Source: CAD feature listing. Evaluate the final solid. Frame: model axes, mm. Coordinates: 2 decimals unless noted, no trailing zeros. Loops run counter-clockwise (first coordinate to the right, second up) from the corner with the lowest first, then second, coordinate; pieces in that order, holes last. Notation, with made-up numbers: M 24,26 L 59,26 A19 cw 59,39 Z; hole C 14.25,-6.75 d5. An arc over 180 degrees is marked long. One line per question, with ' | ' between items. Start each with the question number.
1. Section query A-A, the plane x = 31.75. Output: boundary loops of the cut face in (y, z) (3 decimals).
2. Ray query, probe 1 along X at (y, z) = (5.5, -19.05) (3 decimals); probe 2 along X at (y, z) = (5, 19); probe 3 along Z at (x, y) = (-31, 10). Return the intervals inside material, ascending.
3. Mould query, pull axis Z, two halves, no side actions, for faces 1 (the flat face through (0, 50.8, 0)), 2 (the flat face through (-1, 6, 31.75)), 3 (the cylindrical face through (-34.85, 6.39, -19.74)). Classes: pulls with the +Z half, pulls with the -Z half, needs draft (parallel to the pull), parting line crosses it, or undercut.
4. Pin query (flat end, axial travel): P1, Ø10.5, axis at x = 31.75, z = -19.05, coming from the -Y side; P2, Ø12, axis at y = 28.5, z = 3, coming from the -X side; P3, Ø1, axis at x = 8.5, y = 19.5, coming from the +Z side; P4, Ø7.5, axis at x = -31.75, z = 19.05, coming from the +Y side. Return the tip coordinate at first contact, or that it passes through.
5. Section query D-D, the plane z = 0. Output: boundary loops of the cut face in (x, y).
6. Section query C-C, the plane y = 7. Output: boundary loops of the cut face in (x, z) (3 decimals), and give its area (3 significant figures).
7. Section query B-B, the plane z = 19.05. Output: boundary loops of the cut face in (x, y) (3 decimals).
```python
from build123d import *

# Parameters (mm, degrees)
SKETCH1_W           = 101.6
SKETCH1_H           = 63.5
SKETCH1_R           = 3.175
SKETCH1_R_2         = 3.349234597
BOSS_EXTRUDE1_DEPTH = 12.7
SKETCH2_R           = 12.7
BOSS_EXTRUDE2_DEPTH = 38.1
CHAMFER1_SIZE       = 3.81
FILLET1_R           = 5.08
CHAMFER2_SIZE       = 0.254


with BuildPart() as part:
    # Sketch1 → Boss-Extrude1 (new body)
    with BuildSketch(Plane(origin=(0, 0, 0), x_dir=(1, 0, 0), z_dir=(0, 1, 0))):
        Rectangle(SKETCH1_W, SKETCH1_H)
        with Locations(Location((-31.75, 19.05, 0), (0, 0, 270))):
            Circle(SKETCH1_R, mode=Mode.SUBTRACT)
        with Locations(Location((-31.75, -19.05, 0), (0, 0, 270))):
            Circle(SKETCH1_R, mode=Mode.SUBTRACT)
        with Locations(Location((31.75, -19.05, 0), (0, 0, 270))):
            Circle(SKETCH1_R, mode=Mode.SUBTRACT)
        with Locations(Location((31.75, 19.05, 0), (0, 0, 270))):
            Circle(SKETCH1_R_2, mode=Mode.SUBTRACT)
    extrude(amount=BOSS_EXTRUDE1_DEPTH)

    # Sketch2 → Boss-Extrude2 (add)
    with BuildSketch(Plane(origin=(0, 12.7, 0), x_dir=(1, 0, 0), z_dir=(0, 1, 0))):
        with Locations(Location((0, 0, 0), (0, 0, 90))):
            Circle(SKETCH2_R)
    extrude(amount=BOSS_EXTRUDE2_DEPTH)

    # Chamfer1
    chamfer1_edges = [part.edges().sort_by_distance(p)[0] for p in [
        (0, 12.7, 12.7),
    ]]
    chamfer(chamfer1_edges, length=CHAMFER1_SIZE)

    # Fillet1
    fillet1_edges = [part.edges().sort_by_distance(p)[0] for p in [
        (50.8, 6.35, 31.75),
        (-50.8, 6.35, 31.75),
        (-50.8, 6.35, -31.75),
        (50.8, 6.35, -31.75),
    ]]
    fillet(fillet1_edges, radius=FILLET1_R)

    # Chamfer2
    chamfer2_edges = [part.edges().sort_by_distance(p)[0] for p in [
        (-31.75, 0, 15.875),
        (-31.75, 0, -22.225),
        (31.75, 0, 15.875),
        (31.75, 0, -22.399234597),
        (0, 0, 31.75),
        (50.8, 0, 0),
        (-50.8, 0, 0),
        (0, 0, -31.75),
        (-49.312102448, 0, -30.262102448),
        (49.312102448, 0, -30.262102448),
        (49.312102448, 0, 30.262102448),
        (-49.312102448, 0, 30.262102448),
    ]]
    chamfer(chamfer2_edges, length=CHAMFER2_SIZE)


solid = part.part
```
Taken from the geometry:
1) outline: M 0,-31.496 L 0.254,-31.75 L 12.7,-31.75 L 12.7,-22.399 L 0.254,-22.399 L 0,-22.653 Z; M 0,-15.447 L 0.254,-15.701 L 12.7,-15.701 L 12.7,15.875 L 0.254,15.875 L 0,15.621 Z; M 0,22.479 L 0.254,22.225 L 12.7,22.225 L 12.7,31.75 L 0.254,31.75 L 0,31.496 Z
2) probe 1: -50.8 to -34.925, -28.575 to 28.401, 35.099 to 50.8 | probe 2: -50.8 to -34.92, -28.58 to 28.58, 34.92 to 50.8 | probe 3: -31.75 to -22.14, -15.96 to 15.96, 22.14 to 31.75
3) face 1: needs draft | face 2: pulls with the +Z half | face 3: undercut
4) P1: y = 0 | P2: x = -12.7 | P3: z = 9.86 | P4: y = 12.7
5) outline: M -50.8,0.25 L -50.55,0 L 50.55,0 L 50.8,0.25 L 50.8,12.7 L 16.51,12.7 L 12.7,16.51 L 12.7,50.8 L -12.7,50.8 L -12.7,16.51 L -16.51,12.7 L -50.8,12.7 Z
6) outline: M -50.8,-26.67 A5.08 ccw -45.72,-31.75 L 45.72,-31.75 A5.08 ccw 50.8,-26.67 L 50.8,26.67 A5.08 ccw 45.72,31.75 L -45.72,31.75 A5.08 ccw -50.8,26.67 Z; hole C -31.75,-19.05 d6.35; hole C -31.75,19.05 d6.35; hole C 31.75,-19.05 d6.698; hole C 31.75,19.05 d6.35 | area: 6,300 mm^2
7) outline: M -50.8,0.254 L -50.546,0 L -35.179,0 L -34.925,0.254 L -34.925,12.7 L -50.8,12.7 Z; M -28.575,0.254 L -28.321,0 L 28.321,0 L 28.575,0.254 L 28.575,12.7 L -28.575,12.7 Z; M 34.925,0.254 L 35.179,0 L 50.546,0 L 50.8,0.254 L 50.8,12.7 L 34.925,12.7 Z
